The listing builds one solid part. Answer for the finished solid, in the listing's coordinates (mm). Round coordinates to 2 decimals unless told otherwise and drop trailing zeros. Write each loop counter-clockwise with the first axis right and the second up, starting at its lowest first coordinate (ties: lowest second). Pieces come first, ordered by that corner, then holes. Notation, with made-up numbers: M 12,7 L 63,7 A21 cw 63,28 Z; hole C -11.5,24 d7. An arc over 180 degrees is marked long. One line per item, written item: value. Start each with the question number.
(1) Section A-A (x = 0) is taken. Determine the outline of the cut face in (y, z), plus the area to 3 significant figures.
(2) Section C-C (y = 0) is taken. Determine the outline of the cut face in (x, z), plus the area to 3 significant figures.
(3) Section B-B (z = -3) is taken. Determine the outline of the cut face in (x, y).
(4) Given P1, Ø1.5, axis at x = 1, y = -0.5, coming from the -Z side; P2, Ø1.6, axis at x = 2.93, y = -19.61, coming from the -Z side; P3, Ø3, axis at x = -12, z = 1.5, coming from the -Y side; P4, Ø4.5, axis at y = -14.5, z = 2, coming from the -X side, each flat-ended and moving along its own axis, determine where each tip first touches the part or whether it passes through.
(5) Section D-D (y = 15) is taken. State how many separate pieces and enclosed holes the cut face has, plus the area to 3 significant figures.
(6) For a pull along Y with two mould halves and no side action, classify faces 1 (the cylindrical face through (5.54, -2.3, -2.96)), 2 (the flat face through (5, -19.606, 2)) as released by +Y, released by -Y, zero draft, split by the parting line, or undercut.
(7) Consider probe 1 along Y at (x, z) = (4.5, 3.5); probe 2 along X at (y, z) = (-12.5, 1.5); probe 3 along Y at (x, z) = (3, 3). Determine where each line is inside the solid, lowest interval first.
```python
from build123d import *

# Parameters (mm, degrees)
F0_R             = 30
F0_R_2           = 6
F1_DEPTH         = 4
F2_DEPTH         = 6
F3_R             = 1.5
F4_DEPTH         = 13
F5_W             = 4.6
F5_H             = 3
F6_DEPTH         = 9.4
F11_DEPTH        = 5
F11_COPIES_COUNT = 4


# Not quite as in the source:
# - a pattern or mirror of a feature is missing from the dataset's text; its kind, count and spacing are read off the source's solid


with BuildPart() as f1:
    # F0 (on Top) → F1 (new body)
    with BuildSketch(Plane.XY):
        Circle(F0_R)
        Circle(F0_R_2, mode=Mode.SUBTRACT)
        Circle(F0_R_2)
    extrude(amount=F1_DEPTH)

    # F0 (on Top) → F2 (join)
    with BuildSketch(Plane.XY):
        Circle(F0_R_2)
    extrude(amount=-F2_DEPTH)

    # F3 (on Front) → F4 (cut, symmetric)
    with BuildSketch(Plane.XZ):
        with Locations((0, -3)):
            Circle(F3_R)
    extrude(amount=F4_DEPTH, both=True, mode=Mode.SUBTRACT)

    # F5 (on face) → F6 (cut)
    with BuildSketch(Plane(origin=(0, 0, -6), x_dir=(1, 0, 0), z_dir=(0, 0, -1))):
        with BuildLine():
            ThreePointArc((2.3, -1.5), (2.7459060435, 0), (2.3, 1.5))
            Line((2.3, 1.5), (2.3, -1.5))
        make_face()
        Rectangle(F5_W, F5_H)
        with BuildLine():
            Line((-2.3, -1.5), (-2.3, 1.5))
            ThreePointArc((-2.3, 1.5), (-2.7459060435, 0), (-2.3, -1.5))
        make_face()
    extrude(amount=-F6_DEPTH, mode=Mode.SUBTRACT)

    # F7 (on Front) → F9 (revolve, cut)
    with BuildSketch(Plane.XZ):
        Polygon((-30, 3.3777931239), (-30, 0.5493659992), (-28.5857864376, 1.9635795616), align=None)
    revolve(axis=Axis((0, 0, -3.6810841411), (0, 0, 1)), mode=Mode.SUBTRACT)

    # F10 (on face) → F11 (cut, symmetric)
    with BuildSketch(Plane.XY):
        with BuildLine():
            Line((5.6645294234, 8.9638868584), (5.6645294234, 19.6055186455))
            Line((5.6645294234, 19.6055186455), (3.9258744954, 19.6055186455))
            ThreePointArc((3.9258744954, 19.6055186455), (3.6329812765, 18.8984118643), (2.9258744954, 18.6055186455))
            Line((2.9258744954, 18.6055186455), (2.9258744954, 9.9638868584))
            ThreePointArc((2.9258744954, 9.9638868584), (3.6329812765, 9.6709936396), (3.9258744954, 8.9638868584))
            Line((3.9258744954, 8.9638868584), (5.6645294234, 8.9638868584))
        make_face()
        with BuildLine():
            Line((-2.9258744954, 9.9638868584), (-2.9258744954, 18.6055186455))
            ThreePointArc((-2.9258744954, 18.6055186455), (-3.6329812765, 18.8984118643), (-3.9258744954, 19.6055186455))
            Line((-3.9258744954, 19.6055186455), (-5.6645294234, 19.6055186455))
            Line((-5.6645294234, 19.6055186455), (-5.6645294234, 8.9638868584))
            Line((-5.6645294234, 8.9638868584), (-3.9258744954, 8.9638868584))
            ThreePointArc((-3.9258744954, 8.9638868584), (-3.6329812765, 9.6709936396), (-2.9258744954, 9.9638868584))
        make_face()
        with BuildLine():
            ThreePointArc((2.9258744954, 18.6055186455), (3.6329812765, 18.8984118643), (3.9258744954, 19.6055186455))
            Line((3.9258744954, 19.6055186455), (2.9258744954, 19.6055186455))
            Line((2.9258744954, 19.6055186455), (2.9258744954, 18.6055186455))
        make_face()
        with BuildLine():
            Line((2.9258744954, 18.6055186455), (2.9258744954, 19.6055186455))
            Line((2.9258744954, 19.6055186455), (1.9258744954, 19.6055186455))
            ThreePointArc((1.9258744954, 19.6055186455), (2.2187677142, 18.8984118643), (2.9258744954, 18.6055186455))
        make_face()
        with BuildLine():
            Line((-2.9258744954, 18.6055186455), (-2.9258744954, 19.6055186455))
            Line((-2.9258744954, 19.6055186455), (-3.9258744954, 19.6055186455))
            ThreePointArc((-3.9258744954, 19.6055186455), (-3.6329812765, 18.8984118643), (-2.9258744954, 18.6055186455))
        make_face()
        with BuildLine():
            Line((2.9258744954, 8.9638868584), (3.9258744954, 8.9638868584))
            ThreePointArc((3.9258744954, 8.9638868584), (3.6329812765, 9.6709936396), (2.9258744954, 9.9638868584))
            Line((2.9258744954, 9.9638868584), (2.9258744954, 8.9638868584))
        make_face()
        with BuildLine():
            ThreePointArc((-2.9258744954, 18.6055186455), (-2.2187677142, 18.8984118643), (-1.9258744954, 19.6055186455))
            Line((-1.9258744954, 19.6055186455), (-2.9258744954, 19.6055186455))
            Line((-2.9258744954, 19.6055186455), (-2.9258744954, 18.6055186455))
        make_face()
        with BuildLine():
            Line((-2.9258744954, 8.9638868584), (-2.9258744954, 9.9638868584))
            ThreePointArc((-2.9258744954, 9.9638868584), (-3.6329812765, 9.6709936396), (-3.9258744954, 8.9638868584))
            Line((-3.9258744954, 8.9638868584), (-2.9258744954, 8.9638868584))
        make_face()
        with BuildLine():
            Line((2.9258744954, 8.9638868584), (2.9258744954, 9.9638868584))
            ThreePointArc((2.9258744954, 9.9638868584), (2.2187677142, 9.6709936396), (1.9258744954, 8.9638868584))
            Line((1.9258744954, 8.9638868584), (2.9258744954, 8.9638868584))
        make_face()
        with BuildLine():
            Line((-2.9258744954, 8.9638868584), (-1.9258744954, 8.9638868584))
            ThreePointArc((-1.9258744954, 8.9638868584), (-2.2187677142, 9.6709936396), (-2.9258744954, 9.9638868584))
            Line((-2.9258744954, 9.9638868584), (-2.9258744954, 8.9638868584))
        make_face()
        with BuildLine():
            Line((2.9258744954, 19.6055186455), (3.9258744954, 19.6055186455))
            ThreePointArc((3.9258744954, 19.6055186455), (3.6329812765, 20.3126254267), (2.9258744954, 20.6055186455))
            Line((2.9258744954, 20.6055186455), (2.9258744954, 19.6055186455))
        make_face()
        with BuildLine():
            Line((1.9258744954, 19.6055186455), (2.9258744954, 19.6055186455))
            Line((2.9258744954, 19.6055186455), (2.9258744954, 20.6055186455))
            ThreePointArc((2.9258744954, 20.6055186455), (2.2187677142, 20.3126254267), (1.9258744954, 19.6055186455))
        make_face()
        with BuildLine():
            Line((-2.9258744954, 19.6055186455), (-1.9258744954, 19.6055186455))
            ThreePointArc((-1.9258744954, 19.6055186455), (-2.2187677142, 20.3126254267), (-2.9258744954, 20.6055186455))
            Line((-2.9258744954, 20.6055186455), (-2.9258744954, 19.6055186455))
        make_face()
        with BuildLine():
            Line((-3.9258744954, 19.6055186455), (-2.9258744954, 19.6055186455))
            Line((-2.9258744954, 19.6055186455), (-2.9258744954, 20.6055186455))
            ThreePointArc((-2.9258744954, 20.6055186455), (-3.6329812765, 20.3126254267), (-3.9258744954, 19.6055186455))
        make_face()
        with BuildLine():
            ThreePointArc((-2.9258744954, 7.9638868584), (-2.2187677142, 8.2567800773), (-1.9258744954, 8.9638868584))
            Line((-1.9258744954, 8.9638868584), (-2.9258744954, 8.9638868584))
            Line((-2.9258744954, 8.9638868584), (-2.9258744954, 7.9638868584))
        make_face()
        with BuildLine():
            Line((2.9258744954, 7.9638868584), (2.9258744954, 8.9638868584))
            Line((2.9258744954, 8.9638868584), (1.9258744954, 8.9638868584))
            ThreePointArc((1.9258744954, 8.9638868584), (2.2187677142, 8.2567800773), (2.9258744954, 7.9638868584))
        make_face()
        with BuildLine():
            ThreePointArc((2.9258744954, 7.9638868584), (3.6329812765, 8.2567800773), (3.9258744954, 8.9638868584))
            Line((3.9258744954, 8.9638868584), (2.9258744954, 8.9638868584))
            Line((2.9258744954, 8.9638868584), (2.9258744954, 7.9638868584))
        make_face()
        with BuildLine():
            Line((-2.9258744954, 7.9638868584), (-2.9258744954, 8.9638868584))
            Line((-2.9258744954, 8.9638868584), (-3.9258744954, 8.9638868584))
            ThreePointArc((-3.9258744954, 8.9638868584), (-3.6329812765, 8.2567800773), (-2.9258744954, 7.9638868584))
        make_face()
    f11 = extrude(amount=F11_DEPTH, both=True, mode=Mode.SUBTRACT)

    # F11_copies: F11 ×4 about axis
    f11_copies_axis = Axis((0, 0, 0), (0, 0, 1))
    for i in range(1, F11_COPIES_COUNT):
        add(f11.rotate(f11_copies_axis, i * 360 / F11_COPIES_COUNT), mode=Mode.SUBTRACT)


solid = f1.part
```
Recorded:
1. outline: M -30,0 L -6,0 L -6,-1.5 L -1.5,-1.5 L -1.5,3.4 L 1.5,3.4 L 1.5,-1.5 L 6,-1.5 L 6,0 L 30,0 L 30,0.55 L 28.59,1.96 L 30,3.38 L 30,4 L -30,4 L -30,3.38 L -28.59,1.96 L -30,0.55 Z; M -6,-6 L -1.5,-6 L -1.5,-4.5 L -6,-4.5 Z; M 1.5,-6 L 6,-6 L 6,-4.5 L 1.5,-4.5 Z
1. area: 253 mm2
2. outline: M -30,0 L -6,0 L -6,-6 L -2.75,-6 L -2.75,3.4 L 2.75,3.4 L 2.75,-6 L 6,-6 L 6,0 L 30,0 L 30,0.55 L 28.59,1.96 L 30,3.38 L 30,4 L -30,4 L -30,3.38 L -28.59,1.96 L -30,0.55 Z
2. area: 256 mm2
3. outline: M -2.3,-1.5 A2.75 cw -2.3,1.5 L -1.5,1.5 L -1.5,5.81 A6 ccw -1.5,-5.81 L -1.5,-1.5 Z; M 1.5,-5.81 A6 ccw 1.5,5.81 L 1.5,1.5 L 2.3,1.5 A2.75 cw 2.3,-1.5 L 1.5,-1.5 Z
4. P1: stops at z = 3.4
4. P2: passes through
4. P3: stops at y = -27.97
4. P4: stops at x = -27.17
5. separate pieces: 3
5. enclosed holes: 0
5. area: 181 mm2
6. face 1: split by the parting line
6. face 2: undercut
7. probe 1: y = -29.66 to -19.61, -8.96 to 8.96, 19.61 to 29.66
7. probe 2: x = -26.22 to -5.66, -2.93 to 2.93, 5.66 to 26.22
7. probe 3: y = -29.47 to -20.6, -7.97 to 7.97, 20.6 to 29.47
